```python
from build123d import *

# Parameters (mm, degrees)
F1_DEPTH  = 20
F2_R      = 5
F3_R      = 5
F10_DEPTH = 10
F9_W      = 256
F9_H      = 5
F12_DEPTH = 5
F13_R     = 5


with BuildPart() as f1:
    # F0 (on Front) → F1 (new body)
    with BuildSketch(Plane.XZ):
        with BuildLine():
            ThreePointArc((-71.9452356547, 3.7722354652), (-93.1584390903, 12.5590320296), (-101.9452356547, 33.7722354652))
            Line((-101.9452356547, 33.7722354652), (-141.9452356547, 33.7722354652))
            Line((-141.9452356547, 33.7722354652), (-141.9452356547, -61.2277645348))
            Line((-141.9452356547, -61.2277645348), (128.0547643453, -61.2277645348))
            Line((128.0547643453, -61.2277645348), (128.0547643453, 33.7722354652))
            Line((128.0547643453, 33.7722354652), (88.0547643453, 33.7722354652))
            ThreePointArc((88.0547643453, 33.7722354652), (79.2679677809, 12.5590320296), (58.0547643453, 3.7722354652))
            Line((58.0547643453, 3.7722354652), (-71.9452356547, 3.7722354652))
        make_face()
    extrude(amount=F1_DEPTH)

    # F2
    f2_edges = [f1.edges().sort_by_distance(p)[0] for p in [
        (-101.945236, -10, 33.772235),
    ]]
    fillet(f2_edges, radius=F2_R)

    # F3
    f3_edges = [f1.edges().sort_by_distance(p)[0] for p in [
        (88.054764, -10, 33.772235),
    ]]
    fillet(f3_edges, radius=F3_R)

    # F4 (on face) → F10 (cut)
    with BuildSketch(Plane(origin=(-141.9452356547, 0, 0), x_dir=(0, -1, 0), z_dir=(-1, 0, 0))):
        Polygon((0, -31.2277645348), (0, -41.2277645348), (15, -46.2277645348), (15, -26.2277645348), align=None)
        Polygon((0, 13.7722354652), (0, 3.7722354652), (15, -1.2277645348), (15, 18.7722354652), align=None)
    extrude(amount=-F10_DEPTH, mode=Mode.SUBTRACT)

    # F11: F1 across plane


with BuildPart() as f1_1:
    add(f1.part)
    add(f1.part.mirror(Plane(origin=(-6.9452356547, 0, 3.7722354652), x_dir=(0, 0, -1), z_dir=(1, 0, 0))), mode=Mode.INTERSECT)

    # F9 (on face) → F12 (cut)
    with BuildSketch(Plane(origin=(0, 0, 0), x_dir=(-1, 0, 0), z_dir=(0, 1, 0))):
        with Locations((6.9452356547, -53.7277645348)):
            Rectangle(F9_W, F9_H)
    extrude(amount=-F12_DEPTH, mode=Mode.SUBTRACT)

    # F13
    f13_edges = [f1_1.edges().sort_by_distance(p)[0] for p in [
        (-6.945236, -20, 3.772235),
        (-91.584846, -20, 11.094367),
        (77.694374, -20, 11.094367),
        (-103.312983, -20, 32.55188),
        (89.422512, -20, 32.55188),
        (110.375272, -20, 33.772235),
        (-124.265744, -20, 33.772235),
    ]]
    fillet(f13_edges, radius=F13_R)


solid = f1_1.part
```
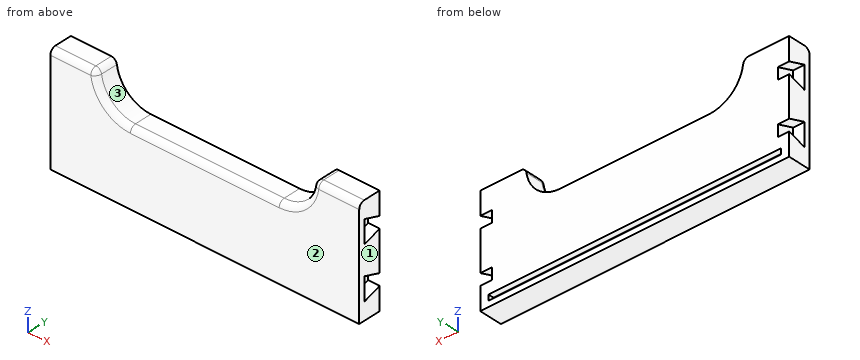
Could you check a few things on this model? Use its own coordinates, in mm. Face numbers are marked on the shaded views. Round coordinates to 2 decimals unless told otherwise and drop trailing zeros. Loops run counter-clockwise (first coordinate to the right, second up) from the corner with the lowest first, then second, coordinate; pieces in that order, holes last.
Q1. I want a section at C-C (x = -60). Write out the boundary of the cut face in (y, z), and give its area (3 significant figures).
Q2. I want a section at A-A (x = -114.5). Write out the boundary of the cut face in (y, z).
Q3. Please list where these lines run through material, in increasing order: L1, parallel to Z at x = -126.5, y = -4.5; L2, parallel to Z at x = 38, y = -11.75; L3, parallel to X at y = -3.5, z = -37.
Q4. I want a section at B-B (y = -17.5). Write out the boundary of the cut face in (x, z), and give its area (3 significant figures).
Q5. For P1, Ø5, axis at x = -135.5, z = -35.5, coming from the +Y side; P2, Ø4, axis at x = -38, z = -53.5, coming from the +Y side; P3, Ø4.5, axis at y = -6, z = -33, coming from the -X side, each with a flat end and sliding along its axis, tell me the tip position at first contact or that it passes through.
Q6. Thinking about a two-plate mould opening in X: for the marked faces 1, 2 and 3, which applies, pulls with the +X half, pulls with the -X half, needs draft (parallel to the pull), parting line crosses it, or undercut?
Answer below:
1. outline: (-20, -61.23) - (0, -61.23) - (0, -56.23) - (-5, -56.23) - (-5, -51.23) - (0, -51.23) - (0, 3.77) - (-15, 3.77) arc R5 ccw to (-20, -1.23) - close
1. area: 1,270 mm2
2. outline: (-20, -61.23) - (0, -61.23) - (0, -56.23) - (-5, -56.23) - (-5, -51.23) - (0, -51.23) - (0, 33.77) - (-15, 33.77) arc R5 ccw to (-20, 28.77) - close
3. L1: z = -61.23 to -56.23, -51.23 to 33.77
3. L2: z = -61.23 to 3.77
3. L3: x = -131.95 to 118.05
4. outline: (-141.95, -61.23) - (128.05, -61.23) - (128.05, 33.1) - (92.7, 33.1) arc R4.33 ccw to (88.41, 29.39) arc R30.67 cw to (58.05, 3.1) - (-71.95, 3.1) arc R30.67 cw to (-102.3, 29.39) arc R4.33 ccw to (-106.59, 33.1) - (-141.95, 33.1) - close
4. area: 20,100 mm2
5. P1: stops at y = -15
5. P2: stops at y = -5
5. P3: stops at x = -131.95
6. face 1: pulls with the +X half
6. face 2: needs draft
6. face 3: undercut
